from build123d import *

# Parameters (mm, degrees)
F0_R     = 40
F1_DEPTH = 2.5


with BuildPart() as f1:
    # F0 (on Front) → F1 (new body, symmetric)
    with BuildSketch(Plane.XZ):
        Circle(F0_R)
        with BuildLine():
            Line((-29.580399, -5), (-5.59017, -5))
            ThreePointArc((-5.59017, -5), (-5.303301, -5.303301), (-5, -5.59017))
            Line((-5, -5.59017), (-5, -29.580399))
            ThreePointArc((-5, -29.580399), (-21.213203, -21.213203), (-29.580399, -5))
        make_face(mode=Mode.SUBTRACT)
        with BuildLine():
            Line((5, -29.580399), (5, -5.59017))
            ThreePointArc((5, -5.59017), (5.303301, -5.303301), (5.59017, -5))
            Line((5.59017, -5), (29.580399, -5))
            ThreePointArc((29.580399, -5), (21.213203, -21.213203), (5, -29.580399))
        make_face(mode=Mode.SUBTRACT)
        with BuildLine():
            Line((-5, 29.580399), (-5, 5.59017))
            ThreePointArc((-5, 5.59017), (-5.303301, 5.303301), (-5.59017, 5))
            Line((-5.59017, 5), (-29.580399, 5))
            ThreePointArc((-29.580399, 5), (-21.213203, 21.213203), (-5, 29.580399))
        make_face(mode=Mode.SUBTRACT)
        with BuildLine():
            ThreePointArc((0, -2.5), (-1.767767, 1.767767), (2.5, 0))
            ThreePointArc((2.5, 0), (1.767767, -1.767767), (0, -2.5))
        make_face(mode=Mode.SUBTRACT)
        with BuildLine():
            ThreePointArc((5, 29.580399), (21.213203, 21.213203), (29.580399, 5))
            Line((29.580399, 5), (5.59017, 5))
            ThreePointArc((5.59017, 5), (5.303301, 5.303301), (5, 5.59017))
            Line((5, 5.59017), (5, 29.580399))
        make_face(mode=Mode.SUBTRACT)
    extrude(amount=F1_DEPTH, both=True)


solid = f1.part
Work out the finished part from the listing and answer in its coordinate system (mm). A direction names the side the tool comes from. Round coordinates to 2 decimals unless told otherwise and drop trailing zeros. Loops run counter-clockwise (first coordinate to the right, second up) from the corner with the lowest first, then second, coordinate; pieces in that order, holes last. Notation, with made-up numbers: (-14.75, 0) -> (1.25, 0) arc R28 cw to (1.25, 26) -> close; hole circle Ø5 at (5, -24). An arc over 180 degrees is marked (long way). Use one line per item in the form item = value.
(1) For a pull along Z with two mould halves and no side action, classify faces 3 (the flat face through (-1, -2.5, -8)), 4 (the flat face through (-17, 0, 5)), 5 (the cylindrical face through (-8.67, -0.04, -39.05)) as released by +Z, released by -Z, zero draft, split by the parting line, or undercut.
Answer list:
face_3 = zero draft
face_4 = undercut
face_5 = split by the parting line
(2) Find section B-B on x = 11. Give the vertices of the cut face in (y, z), then the cut area to 3 significant figures.
Answer list:
outline = (-2.5, -38.46) -> (2.5, -38.46) -> (2.5, -27.91) -> (-2.5, -27.91) -> close; (-2.5, -5) -> (2.5, -5) -> (2.5, 5) -> (-2.5, 5) -> close; (-2.5, 27.91) -> (2.5, 27.91) -> (2.5, 38.46) -> (-2.5, 38.46) -> close
area = 155 mm2
(3) Straight lines are drawn through the part: line 1 (X direction, y = -0.4, z = -11.5); line 2 (X direction, y = -1.9, z = 16); line 3 (Z direction, x = -15, y = -2). For each, find the intervals that lie inside material, in ascending order.
Answer list:
line_1 = -38.31 to -27.71, -5 to 5, 27.71 to 38.31
line_2 = -36.66 to -25.38, -5 to 5, 25.38 to 36.66
line_3 = -37.08 to -25.98, -5 to 5, 25.98 to 37.08
(4) Flat-ended cylindrical pins translate along their axes: P1, Ø1, axis at y = -1.5, z = 17.5, coming from the +X side; P2, Ø2.5, axis at y = 0, z = -12, coming from the -X side; P3, Ø1.5, axis at x = -17.5, y = 0, coming from the -Z side. Find the tip coordinate at first contact, or state that the pin passes through.
Answer list:
P1 = 36.21
P2 = -38.53
P3 = -36.32
(5) Find section C-C on z = 14. Give the vertices of the cut face in (x, y).
Answer list:
outline = (-37.47, -2.5) -> (-26.53, -2.5) -> (-26.53, 2.5) -> (-37.47, 2.5) -> close; (-5, -2.5) -> (5, -2.5) -> (5, 2.5) -> (-5, 2.5) -> close; (26.53, -2.5) -> (37.47, -2.5) -> (37.47, 2.5) -> (26.53, 2.5) -> close
(6) Find section A-A on y = -1.65. Give the vertices of the cut face in (x, z).
Answer list:
outline = circle Ø80 at (0, 0); hole (-29.58, -5) arc R30 ccw to (-5, -29.58) -> (-5, -5.59) arc R7.5 cw to (-5.59, -5) -> close; hole (-29.58, 5) -> (-5.59, 5) arc R7.5 cw to (-5, 5.59) -> (-5, 29.58) arc R30 ccw to start; hole circle Ø5 at (0, 0); hole (5, -29.58) arc R30 ccw to (29.58, -5) -> (5.59, -5) arc R7.5 cw to (5, -5.59) -> close; hole (5, 5.59) arc R7.5 cw to (5.59, 5) -> (29.58, 5) arc R30 ccw to (5, 29.58) -> close
(7) Find section D-D on x = 33.5. Give the vertices of the cut face in (y, z).
Answer list:
outline = (-2.5, -21.86) -> (2.5, -21.86) -> (2.5, 21.86) -> (-2.5, 21.86) -> close
(8) A tool of negligible diameter and unlimited length cuts with its end or side. For faces 1 (the cylindrical face through (21.029, -0.035, 21.396)), 2 (the flat face through (-1, 2.5, -8)), from which of +Z, -Z, +X, -X, +Y, -Y can it reach the whole face along a straight path? Write none if from no direction.
Answer list:
face_1 = +Y, -Y
face_2 = +Z, -Z, +X, -X, +Y
